Here's how the part is built. I have some questions about the finished solid (model axes, mm). A direction names the side the tool comes from. Round coordinates to 2 decimals unless told otherwise and drop trailing zeros. Loops run counter-clockwise (first coordinate to the right, second up) from the corner with the lowest first, then second, coordinate; pieces in that order, holes last. Notation, with made-up numbers: M 15.25,-30.75 L 49.25,-30.75 A34 ccw 49.25,-0.75 Z; hole C 20.5,-29 d9. An arc over 180 degrees is marked long. Write item = value, one per line. Start each with the question number.
from build123d import *

# Parameters (mm, degrees)
SKETCH1_W           = 95
SKETCH1_H           = 65
BOSS_EXTRUDE1_DEPTH = 4.2
FILLET1_R           = 10
FILLET2_R           = 4
SHELL1_T            = -1.2
SKETCH5_R           = 4.5
BOSS_EXTRUDE3_DEPTH = 3
SKETCH7_R           = 1.75
CUT_EXTRUDE2_DEPTH  = 10
BOSS_EXTRUDE4_REACH = 117.185
BOSS_EXTRUDE5_DEPTH = 1
BOSS_EXTRUDE5_DRAFT = 10
SKETCH12_R          = 3.5
CUT_EXTRUDE3_DEPTH  = 3
SKETCH13_W          = 23
SKETCH13_H          = 16
CUT_EXTRUDE4_DEPTH  = 116.226038806
FILLET3_R           = 2


with BuildPart() as part:
    # Sketch1 → Boss-Extrude1 (new body)
    with BuildSketch(Plane(origin=(0, 0, 0), x_dir=(1, 0, 0), z_dir=(0, 1, 0))):
        with Locations((47.5, 32.5)):
            Rectangle(SKETCH1_W, SKETCH1_H)
    extrude(amount=BOSS_EXTRUDE1_DEPTH)

    # Fillet1
    fillet1_edges = [part.edges().sort_by_distance(p)[0] for p in [
        (0, 2.1, -65),
        (95, 2.1, -65),
        (95, 2.1, 0),
        (0, 2.1, 0),
    ]]
    fillet(fillet1_edges, radius=FILLET1_R)

    # Fillet2
    fillet2_edges = [part.edges().sort_by_distance(p)[0] for p in [
        (95, 0, -32.5),
        (0, 0, -32.5),
        (47.5, 0, -65),
        (47.5, 0, 0),
        (2.928932188, 0, -2.928932188),
        (2.928932188, 0, -62.071067812),
        (92.071067812, 0, -62.071067812),
        (92.071067812, 0, -2.928932188),
    ]]
    fillet(fillet2_edges, radius=FILLET2_R)

    # Shell1
    shell1_openings = [part.faces().sort_by_distance(p)[0] for p in [
        (47.5, 4.2, -32.5),
    ]]
    offset(amount=SHELL1_T, openings=shell1_openings, kind=Kind.INTERSECTION)

    # Sketch5 → Boss-Extrude3 (add)
    with BuildSketch(Plane(origin=(0, 1.2, 0), x_dir=(1, 0, 0), z_dir=(0, 1, 0))):
        with Locations(Location((10, 55, 0), (0, 0, 90))):
            Circle(SKETCH5_R)
        with Locations(Location((85, 55, 0), (0, 0, 90))):
            Circle(SKETCH5_R)
        with Locations(Location((85, 10, 0), (0, 0, 90))):
            Circle(SKETCH5_R)
        with Locations(Location((10, 10, 0), (0, 0, 90))):
            Circle(SKETCH5_R)
    extrude(amount=BOSS_EXTRUDE3_DEPTH)

    # Sketch7 → Cut-Extrude2 (cut)
    with BuildSketch(Plane(origin=(0, 4.2, 0), x_dir=(1, 0, 0), z_dir=(0, 1, 0))):
        with Locations(Location((10, 55, 0), (0, 0, 270))):
            Circle(SKETCH7_R)
        with Locations(Location((85, 55, 0), (0, 0, 270))):
            Circle(SKETCH7_R)
        with Locations(Location((85, 10, 0), (0, 0, 270))):
            Circle(SKETCH7_R)
        with Locations(Location((10, 10, 0), (0, 0, 270))):
            Circle(SKETCH7_R)
    extrude(amount=-CUT_EXTRUDE2_DEPTH, mode=Mode.SUBTRACT)

    # Sketch8 → Boss-Extrude4 (add, up to next)
    with BuildSketch(Plane(origin=(0, 4.2, 0), x_dir=(1, 0, 0), z_dir=(0, 1, 0)), mode=Mode.PRIVATE) as boss_extrude4_sk1:
        with BuildLine():
            Line((1.2, 55), (1.2, 10))
            ThreePointArc((1.2, 10), (3.777460326, 3.777460326), (10, 1.2))
            Line((10, 1.2), (85, 1.2))
            ThreePointArc((85, 1.2), (91.222539674, 3.777460326), (93.8, 10))
            Line((93.8, 10), (93.8, 55))
            ThreePointArc((93.8, 55), (91.222539674, 61.222539674), (85, 63.8))
            Line((85, 63.8), (10, 63.8))
            ThreePointArc((10, 63.8), (3.777460326, 61.222539674), (1.2, 55))
        make_face()
        with BuildLine():
            Line((85, 62.8), (10, 62.8))
            ThreePointArc((10, 62.8), (4.484567107, 60.515432893), (2.2, 55))
            Line((2.2, 55), (2.2, 10))
            ThreePointArc((2.2, 10), (4.484567107, 4.484567107), (10, 2.2))
            Line((10, 2.2), (85, 2.2))
            ThreePointArc((85, 2.2), (90.515432893, 4.484567107), (92.8, 10))
            Line((92.8, 10), (92.8, 55))
            ThreePointArc((92.8, 55), (90.515432893, 60.515432893), (85, 62.8))
        make_face(mode=Mode.SUBTRACT)
    boss_extrude4_tool1 = extrude(boss_extrude4_sk1.sketch, amount=-BOSS_EXTRUDE4_REACH, mode=Mode.PRIVATE) - part.part
    add(boss_extrude4_tool1.solids().sort_by_distance((1.311774, 4.2, -32.5))[0])


with BuildPart() as boss_extrude5_tool:
    # Sketch11 → Boss-Extrude5 (with draft: the straight prism first)
    with BuildSketch(Plane(origin=(0, 4.2, 0), x_dir=(1, 0, 0), z_dir=(0, 1, 0))):
        with BuildLine():
            Line((93.6, 10), (93.6, 55))
            ThreePointArc((93.6, 55), (91.081118318, 61.081118318), (85, 63.6))
            Line((85, 63.6), (10, 63.6))
            ThreePointArc((10, 63.6), (3.918881682, 61.081118318), (1.4, 55))
            Line((1.4, 55), (1.4, 10))
            ThreePointArc((1.4, 10), (3.918881682, 3.918881682), (10, 1.4))
            Line((10, 1.4), (85, 1.4))
            ThreePointArc((85, 1.4), (91.081118318, 3.918881682), (93.6, 10))
        make_face()
        with BuildLine():
            Line((92.8, 10), (92.8, 55))
            ThreePointArc((92.8, 55), (90.515432893, 60.515432893), (85, 62.8))
            Line((85, 62.8), (10, 62.8))
            ThreePointArc((10, 62.8), (4.484567107, 60.515432893), (2.2, 55))
            Line((2.2, 55), (2.2, 10))
            ThreePointArc((2.2, 10), (4.484567107, 4.484567107), (10, 2.2))
            Line((10, 2.2), (85, 2.2))
            ThreePointArc((85, 2.2), (90.515432893, 4.484567107), (92.8, 10))
        make_face(mode=Mode.SUBTRACT)
    extrude(amount=BOSS_EXTRUDE5_DEPTH)
    # Boss-Extrude5: the draft: its side faces are tilted about the plane it starts from
    boss_extrude5_sides = [boss_extrude5_tool.faces().sort_by_distance(p)[0] for p in [
        (91.081118318, 4.7, -3.918881682),
        (93.6, 4.7, -32.5),
        (91.081118318, 4.7, -61.081118318),
        (47.5, 4.7, -63.6),
        (3.918881682, 4.7, -61.081118318),
        (1.4, 4.7, -32.5),
        (3.918881682, 4.7, -3.918881682),
        (47.5, 4.7, -1.4),
        (47.5, 4.7, -2.2),
        (4.484567107, 4.7, -4.484567107),
        (2.2, 4.7, -32.5),
        (4.484567107, 4.7, -60.515432893),
        (47.5, 4.7, -62.8),
        (90.515432893, 4.7, -60.515432893),
        (92.8, 4.7, -32.5),
        (90.515432893, 4.7, -4.484567107),
    ]]
    draft(boss_extrude5_sides, Plane(origin=(0, 4.2, 0), x_dir=(1, 0, 0), z_dir=(0, 1, 0)), BOSS_EXTRUDE5_DRAFT)


with BuildPart() as part_1:
    add(part.part)

    # Boss-Extrude5: add boss_extrude5_tool
    add(boss_extrude5_tool.part)

    # Sketch12 → Cut-Extrude3 (cut)
    with BuildSketch(Plane.XZ):
        with Locations(Location((10, -10, 0), (0, 0, 270))):
            Circle(SKETCH12_R)
        with Locations(Location((85, -10, 0), (0, 0, 270))):
            Circle(SKETCH12_R)
        with Locations(Location((85, -55, 0), (0, 0, 270))):
            Circle(SKETCH12_R)
        with Locations(Location((10, -55, 0), (0, 0, 270))):
            Circle(SKETCH12_R)
    extrude(amount=-CUT_EXTRUDE3_DEPTH, mode=Mode.SUBTRACT)

    # Sketch13 → Cut-Extrude4 (cut, through all)
    with BuildSketch(Plane.XZ):
        with Locations((34.5, -32.5)):
            Rectangle(SKETCH13_W, SKETCH13_H)
    extrude(amount=-CUT_EXTRUDE4_DEPTH, mode=Mode.SUBTRACT)

    # Fillet3
    fillet3_edges = [part_1.edges().sort_by_distance(p)[0] for p in [
        (46, 0.6, -24.5),
        (46, 0.6, -40.5),
        (23, 0.6, -40.5),
        (23, 0.6, -24.5),
    ]]
    fillet(fillet3_edges, radius=FILLET3_R)


solid = part_1.part
Item 1: I want a section at B-B, the plane z = -47.5. List the corners of the cut face in (x, y) for me.
Item 2: For faces 1 (the flat face through (12, 3, -11)), 2 (the conical face through (91.07, 4.8, -60.94)), 3 (the flat face through (47, 0, -33)), 4 (the flat face through (92.8, 3, -32)), 5 (the cylindrical face through (45.4, 0.61, -25.07)), which set-ups out of +Z, -Z, +X, -X, +Y, -Y let a thin tool reach every point of the face, with its end or its side?
Item 3: Please list where these lines run through material, in increasing order: line 1 (X direction, y = 3.65, z = -49); line 2 (Z direction, x = 85, y = 3.7); line 3 (X direction, y = 3.3, z = -55). Write a range as [from, to].
Item 4: I want a section at A-A, the plane z = -34.5. List the corners of the cut face in (x, y) for me, then the cut area to 3 significant figures.
Item 5: Will these pins go through, and if not, where does the flat tip stop? pin 1 Ø10 at (x, z) = (85, -11.5) entering from +Y; pin 2 Ø17 at (x, z) = (35.5, -41) entering from +Y; pin 3 Ø5.5 at (x, z) = (10, -55) entering from -Y.
Worked out:
q1.outline = M 0,4 A4 ccw 4,0 L 91,0 A4 ccw 95,4 L 95,4.2 L 93.6,4.2 L 93.42,5.2 L 92.98,5.2 L 92.8,4.2 L 92.8,1.86 A2.8 cw 91,1.2 L 4,1.2 A2.8 cw 2.2,1.86 L 2.2,4.2 L 2.02,5.2 L 1.58,5.2 L 1.4,4.2 L 0,4.2 Z
q2.face_1 = -Y
q2.face_2 = -Z, +X, +Y
q2.face_3 = +Z, -Z, +X, -X, -Y
q2.face_4 = +Y
q2.face_5 = +Y, -Y
q3.line_1 = [0.02, 2.2], [92.8, 94.98]
q3.line_2 = [-64.99, -62.8], [-59.5, -56.75], [-53.25, -50.5], [-14.5, -11.75], [-8.25, -5.5], [-2.2, -0.01]
q3.line_3 = [0.06, 2.2], [5.5, 8.25], [11.75, 14.5], [80.5, 83.25], [86.75, 89.5], [92.8, 94.94]
q4.outline = M 0,4 A4 ccw 4,0 L 23,0 L 23,1.2 L 4,1.2 A2.8 cw 2.2,1.86 L 2.2,4.2 L 2.02,5.2 L 1.58,5.2 L 1.4,4.2 L 0,4.2 Z; M 46,0 L 91,0 A4 ccw 95,4 L 95,4.2 L 93.6,4.2 L 93.42,5.2 L 92.98,5.2 L 92.8,4.2 L 92.8,1.86 A2.8 cw 91,1.2 L 46,1.2 Z
q4.area = 94.7 mm2
q5.pin_1 = 4.2
q5.pin_2 = 1.2
q5.pin_3 = 3
